Verification items for this drawing (mm, ordinates from the low corner). A direction names the side the tool comes from. Give positions to 0.01 mm unless a question says otherwise; leave off trailing zeros. Loops run counter-clockwise (first coordinate to the right, second up) from the corner with the lowest first, then second, coordinate; pieces in that order, holes last. Notation, with made-up numbers: (63.5, 52) -> (81.5, 52) arc R11 cw to (81.5, 68) -> close; hole circle Ø4 at (3, -0.5). An arc over 180 degrees is marked (long way). Answer as CSV lines item,"result". Start each with the question number.
(1) Gauge pin test, flat ends, axial feed: pin 1 Ø2 at (y, z) = (16.5, 2) entering from +X; pin 2 Ø1.5 at (y, z) = (14, 2) entering from -X; pin 3 Ø2 at (y, z) = (11, 4) entering from -X. Record the tip position at first contact, or that the pin passes through.
(2) Material ranges on line 1 (Z direction, x = 6.75, y = 4.25); line 2 (Z direction, x = 6, y = 12.75); line 3 (X direction, y = 16, z = 1.2), recorded low to high. Write a range as from..to.
(3) Section check D-D on z = 1.1. Enter the section's corners in (x, y), plus the area to 3 significant figures.
(4) Section check C-C on z = 2.75. Enter the section's corners in (x, y).
(5) Section check A-A on x = 9.5. Enter the section's corners in (y, z), plus the area to 3 significant figures.
(6) Access from +Z, -Z, +X, -X, +Y, -Y to the whole of each face (thin tool, end or side, straight path). Record for the marked faces 1 and 2.
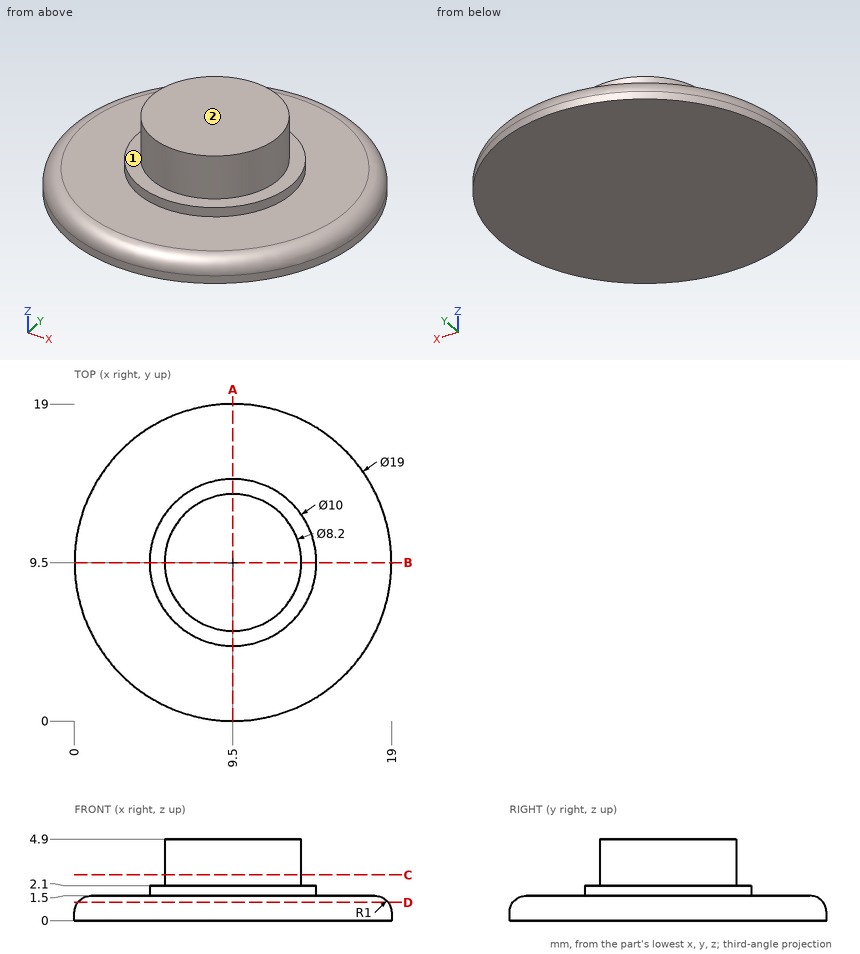
Working result:
1,pin 1,"stops at x = 16.13"
1,pin 2,"stops at x = 1.44"
1,pin 3,"stops at x = 5.43"
2,line 1,"z = 0..1.5"
2,line 2,"z = 0..2.1"
2,line 3,"x = 2.97..16.03"
3,outline,"circle Ø18.6 at (9.5, 9.5)"
3,area,"272 mm^2"
4,outline,"circle Ø8.2 at (9.5, 9.5)"
5,outline,"(0, 0) -> (19, 0) -> (19, 0.5) arc R1 ccw to (18, 1.5) -> (14.5, 1.5) -> (14.5, 2.1) -> (13.6, 2.1) -> (13.6, 4.9) -> (5.4, 4.9) -> (5.4, 2.1) -> (4.5, 2.1) -> (4.5, 1.5) -> (1, 1.5) arc R1 ccw to (0, 0.5) -> close"
5,area,"57.0 mm^2"
6,face 1,"+Z"
6,face 2,"+Z, +X, -X, +Y, -Y"
